from build123d import *

# Parameters (mm, degrees)
SKETCH_1_W          = 55
SKETCH_1_H          = 25
SKETCH_1_R          = 4.435900657
EXTRUDE_1_DEPTH     = 20
SKETCH_2_W          = 6
SKETCH_2_H          = 25
EXTRUDE_2_DEPTH     = 25
SKETCH_3_R          = 2.5
CUT_EXTRUDE_1_DEPTH = 70.564485554


with BuildPart() as part:
    # 草图1 → 凸台-拉伸1 (new body)
    with BuildSketch(Plane.XY):
        with Locations((-22.681333333, 7.827755665)):
            Rectangle(SKETCH_1_W, SKETCH_1_H)
        with Locations((-37.681333333, 7.827755665)):
            Circle(SKETCH_1_R, mode=Mode.SUBTRACT)
        with Locations(Location((-7.681333333, 7.827755665, 0), (0, 0, 180))):
            Circle(SKETCH_1_R, mode=Mode.SUBTRACT)
    extrude(amount=EXTRUDE_1_DEPTH)

    # 草图2 → 凸台-拉伸2 (add)
    with BuildSketch(Plane.XY.offset(20)):
        with Locations((-47.181333333, 7.827755665)):
            Rectangle(SKETCH_2_W, SKETCH_2_H)
    extrude(amount=EXTRUDE_2_DEPTH)

    # 草图3 → 切除-拉伸1 (cut, through all)
    with BuildSketch(Plane(origin=(-44.181333333, 0, 0), x_dir=(0, 0, -1), z_dir=(1, 0, 0))):
        with Locations((-37.5, 2.827755665)):
            Circle(SKETCH_3_R)
        with Locations((-27.5, 12.827755665)):
            Circle(SKETCH_3_R)
    extrude(amount=-CUT_EXTRUDE_1_DEPTH, mode=Mode.SUBTRACT)


solid = part.part
Work out the finished part from the listing and answer in its coordinate system (mm). A direction names the side the tool comes from. Give positions to 0.01 mm unless a question says otherwise; leave off trailing zeros. Loops run counter-clockwise (first coordinate to the right, second up) from the corner with the lowest first, then second, coordinate; pieces in that order, holes last. Notation, with made-up numbers: (28, 72) - (39, 72) arc R18 cw to (39, 102) - close; hole circle Ø2 at (-9, 47.25). An arc over 180 degrees is marked (long way). Answer in a Markdown table with one row per item.
(1) Section D-D (z = 7) is taken. Give the vertices of the cut face in (x, y), and give its area (3 significant figures).
Results list:
| item | result |
|---|---|
| outline | (-50.18, -4.67) - (4.82, -4.67) - (4.82, 20.33) - (-50.18, 20.33) - close; hole circle Ø8.87 at (-37.68, 7.83); hole circle Ø8.87 at (-7.68, 7.83) |
| area | 1,250 mm² |
(2) Section B-B (y = 6) is taken. Give the vertices of the cut face in (x, z).
Results list:
| item | result |
|---|---|
| outline | (-50.18, 0) - (-41.72, 0) - (-41.72, 20) - (-44.18, 20) - (-44.18, 45) - (-50.18, 45) - close; (-33.64, 0) - (-11.72, 0) - (-11.72, 20) - (-33.64, 20) - close; (-3.64, 0) - (4.82, 0) - (4.82, 20) - (-3.64, 20) - close |
(3) Section C-C (x = -39) is taken. Give the vertices of the cut face in (y, z), and give its area (3 significant figures).
Results list:
| item | result |
|---|---|
| outline | (-4.67, 0) - (3.59, 0) - (3.59, 20) - (-4.67, 20) - close; (12.06, 0) - (20.33, 0) - (20.33, 20) - (12.06, 20) - close |
| area | 331 mm² |
(4) Flat-ended cylindrical pins translate along their axes: pin 1 Ø11.5 at (x, y) = (-7.68, 7.83) entering from +Z; pin 2 Ø4 at (y, z) = (11, 24.5) entering from +X; pin 3 Ø1.5 at (x, y) = (-37, 13) entering from -Z. Find the tip coordinate at first contact, or state that the pin passes through.
Results list:
| item | result |
|---|---|
| pin 1 | stops at z = 20 |
| pin 2 | stops at x = -44.18 |
| pin 3 | stops at z = 0 |
(5) Consider L1, parallel to X at y = 8, z = 8; L2, parallel to X at y = 6, z = 10.5; L3, parallel to Z at x = 3.5, y = -2. Determine where each line is inside the solid, lowest interval first. Write a range as [from, to].
Results list:
| item | result |
|---|---|
| L1 | x = [-50.18, -42.11], [-33.25, -12.11], [-3.25, 4.82] |
| L2 | x = [-50.18, -41.72], [-33.64, -11.72], [-3.64, 4.82] |
| L3 | z = [0, 20] |
(6) A tool of negligible diameter and unlimited length cuts with its end or side. For faces 1 (the face through (-44.181, 8, 32)), 2 (the face through (-50.181, 8, 22)), from which of +Z, -Z, +X, -X, +Y, -Y can it reach the whole face along a straight path? Write none if from no direction.
Results list:
| item | result |
|---|---|
| face 1 | +Z, +X, +Y, -Y |
| face 2 | +Z, -Z, -X, +Y, -Y |
(7) Section A-A (z = 37.5) is taken. Give the vertices of the cut face in (x, y), and give its area (3 significant figures).
Results list:
| item | result |
|---|---|
| outline | (-50.18, -4.67) - (-44.18, -4.67) - (-44.18, 0.33) - (-50.18, 0.33) - close; (-50.18, 5.33) - (-44.18, 5.33) - (-44.18, 20.33) - (-50.18, 20.33) - close |
| area | 120 mm² |
(8) For a pull along Y with two mould halves and no side action, classify faces 3 (the face through (-23, 8, 0)), 4 (the face through (-47.14, 1.87, 35.19)), 5 (the face through (-23, -4.672, 12)) as pulls with the +Y half, pulls with the -Y half, needs draft (parallel to the pull), parting line crosses it, or undercut.
Results list:
| item | result |
|---|---|
| face 3 | needs draft |
| face 4 | undercut |
| face 5 | pulls with the -Y half |
